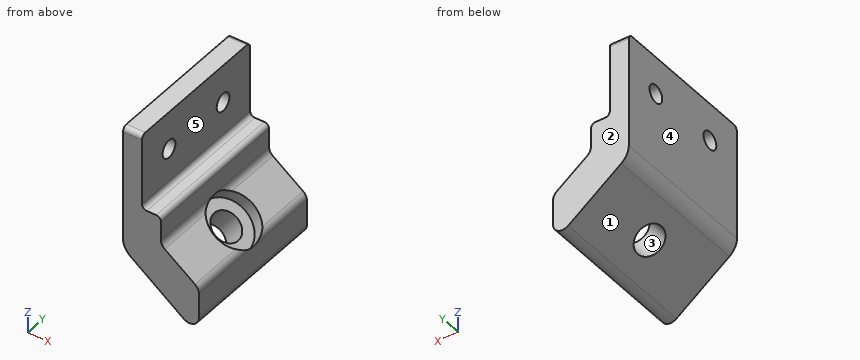
```python
from build123d import *

# Parameters (mm, degrees)
BOSS_EXTRUDE1_DEPTH = 50.8
SKETCH15_R          = 5
CUT_EXTRUDE14_DEPTH = 8.89
SKETCH16_R          = 8.89
CUT_EXTRUDE15_DEPTH = 6.858
SKETCH17_R          = 3
CUT_EXTRUDE16_DEPTH = 6.35


with BuildPart() as part:
    # Sketch1 → Boss-Extrude1 (new body)
    with BuildSketch(Plane(origin=(0, 0, 0), x_dir=(1, 0, 0), z_dir=(0, 1, 0))):
        with BuildLine():
            Line((31.75, 0), (31.75, 13.171631631))
            Line((31.75, 13.171631631), (31.75, 38.571631565))
            ThreePointArc((31.75, 38.571631565), (32.413933313, 41.398493011), (34.266896261, 43.63422139))
            Line((34.266896261, 43.63422139), (52.058448131, 57.104967856))
            ThreePointArc((52.058448131, 57.104967856), (55.388430723, 57.416706287), (57.15, 54.573672944))
            Line((57.15, 54.573672944), (57.15, 46.0375))
            ThreePointArc((57.15, 46.0375), (56.814806331, 44.617596834), (55.88, 43.4975))
            Line((55.88, 43.4975), (45.72, 35.8775))
            ThreePointArc((45.72, 35.8775), (44.785193669, 34.757403166), (44.45, 33.3375))
            Line((44.45, 33.3375), (44.45, 26.9875))
            ThreePointArc((44.45, 26.9875), (43.985032015, 25.864967985), (42.8625, 25.4))
            Line((42.8625, 25.4), (39.6875, 25.4))
            ThreePointArc((39.6875, 25.4), (38.564967985, 24.935032015), (38.1, 23.8125))
            Line((38.1, 23.8125), (38.1, 0))
            Line((38.1, 0), (31.75, 0))
        make_face()
    extrude(amount=-BOSS_EXTRUDE1_DEPTH)

    # Sketch15 → Cut-Extrude14 (cut)
    with BuildSketch(Plane(origin=(-8.51306907, 0, -11.243676088), x_dir=(-0.79725824, 0, 0.603638384), z_dir=(-0.603638384, 0, -0.79725824))):
        with Locations((-64.492331876, -25.4)):
            Circle(SKETCH15_R)
    extrude(amount=-CUT_EXTRUDE14_DEPTH, mode=Mode.SUBTRACT)

    # Sketch16 → Cut-Extrude15 (cut)
    with BuildSketch(Plane(origin=(0.762, 0, 1.016), x_dir=(0.8, 0, -0.6), z_dir=(0.6, 0, 0.8))):
        with Locations((64.467913736, -25.4)):
            Circle(SKETCH16_R)
    extrude(amount=-CUT_EXTRUDE15_DEPTH, mode=Mode.SUBTRACT)

    # Sketch17 → Cut-Extrude16 (cut)
    with BuildSketch(Plane.ZY.offset(-31.75)):
        with Locations((-12.7, -12.7)):
            Circle(SKETCH17_R)
        with Locations((-12.7, -38.1)):
            Circle(SKETCH17_R)
        with BuildLine():
            Line((-1.5875, -50.8), (0, -50.8))
            Line((0, -50.8), (0, -49.2125))
            ThreePointArc((0, -49.2125), (-0.464967985, -50.335032015), (-1.5875, -50.8))
        make_face()
        with BuildLine():
            Line((-1.5875, 0), (0, 0))
            Line((0, 0), (0, -1.5875))
            ThreePointArc((0, -1.5875), (-0.464967985, -0.464967985), (-1.5875, 0))
        make_face()
    extrude(amount=-CUT_EXTRUDE16_DEPTH, mode=Mode.SUBTRACT)


solid = part.part
```
Here's how the part is built. I have some questions about the finished solid (model axes, mm). Face numbers are marked on the shaded views. A direction names the side the tool comes from. Coordinates: 2 decimals unless noted, no trailing zeros. Loops run counter-clockwise (first coordinate to the right, second up) from the corner with the lowest first, then second, coordinate; pieces in that order, holes last. Notation, with made-up numbers: (55.5, 8) - (101.5, 8) arc R10 cw to (101.5, 16) - close; hole circle Ø10 at (-17.5, 20). An arc over 180 degrees is marked (long way). Return JSON: item names as keys, results as strings. Group by question number.
Item 1: If we section it at D-D on z = -32: Write out the boundary of the cut face in (x, y), and give its area (3 significant figures).
Item 2: If we section it at C-C on z = -22.5: Write out the boundary of the cut face in (x, y), and give its area (3 significant figures).
Item 3: On a 3-axis mill with a long thin cutter (end or side, diameter ignored), from which of +Z, -Z, +X, -X, +Y, -Y can I reach the whole of each face in a straight line? I mean the marked faces 4 and 5. Say none if no direction works.
Item 4: We'd pull the mould along Y, two halves only. Please class the marked faces 1, 2 and 3: +Y half, -Y half, draft (parallel to the pull), parting line (faces both ways), or undercut.
Item 5: If we section it at B-B on z = -12.7: Write out the boundary of the cut face in (x, y).
Item 6: Will these pins go through, and if not, where does the flat tip stop? P1, Ø10, axis at x = 44.5, z = -45, coming from the +Y side; P2, Ø8, axis at y = -38.1, z = -12.7, coming from the +X side; P3, Ø1.5, axis at x = 45.5, y = -25.5, coming from the -Z side; P4, Ø1.6, axis at x = 41, y = -22.5, coming from the +Z side.
Item 7: I need wall thicknesses on line 1 (Y direction, x = 34, z = -12.7); line 2 (X direction, y = -27.5, z = -46); line 3 (X direction, y = -22, z = -11.5). Which ranges of each line are inside material? Lowest first, please. Write a range as from..to.
Calculated:
{
 "1": {"outline": "(31.75, -50.8) - (44.45, -50.8) - (44.45, 0) - (31.75, 0) - close", "area": "645 mm^2"},
 "2": {"outline": "(31.75, -50.8) - (38.1, -50.8) - (38.1, 0) - (31.75, 0) - close", "area": "323 mm^2"},
 "3": {"face 4": "+Z, -Z, -X, +Y, -Y", "face 5": "+Z, +X, +Y, -Y"},
 "4": {"face 1": "draft", "face 2": "+Y half", "face 3": "undercut"},
 "5": {"outline": "(31.75, -50.8) - (38.1, -50.8) - (38.1, -41.1) - (31.75, -41.1) - close; (31.75, -35.1) - (38.1, -35.1) - (38.1, -15.7) - (31.75, -15.7) - close; (31.75, -9.7) - (38.1, -9.7) - (38.1, 0) - (31.75, 0) - close"},
 "6": {"P1": "stops at y = 0", "P2": "stops at x = 38.1", "P3": "passes through", "P4": "stops at z = -25.4"},
 "7": {"line 1": "y = -50.8..-41.1, -35.1..-15.7, -9.7..0", "line 2": "x = 37.39..40.37, 51.76..52.02, 56.88..57.15", "line 3": "x = 31.75..38.1"}
}
